```python
from build123d import *

# Parameters (mm, degrees)
F0_R     = 11.949999
F0_R_2   = 5.401318
F1_DEPTH = 25.4
F2_DEPTH = 51.308
F3_R     = 5.08
F4_SIZE  = 5.08


with BuildPart() as f1:
    # F0 (on Front) → F1 (new body)
    with BuildSketch(Plane.XZ):
        with BuildLine():
            ThreePointArc((4.758947, -26.106481), (20.377471, -16.998665), (26.53669, 0))
            ThreePointArc((26.53669, 0), (20.377471, 16.998665), (4.758947, 26.106481))
            ThreePointArc((4.758947, 26.106481), (-26.53669, 0), (4.758947, -26.106481))
        make_face()
        Circle(F0_R, mode=Mode.SUBTRACT)
        with BuildLine():
            ThreePointArc((4.758947, 26.106481), (20.377471, 16.998665), (26.53669, 0))
            ThreePointArc((26.53669, 0), (20.377471, -16.998665), (4.758947, -26.106481))
            Line((4.758947, -26.106481), (78.85573, -12.599387))
            ThreePointArc((78.85573, -12.599387), (63.751977, 0), (78.85573, 12.599387))
            Line((78.85573, 12.599387), (4.758947, 26.106481))
        make_face()
        with BuildLine():
            ThreePointArc((89.366002, 0), (86.393468, 8.203815), (78.85573, 12.599387))
            ThreePointArc((78.85573, 12.599387), (63.751977, 0), (78.85573, -12.599387))
            ThreePointArc((78.85573, -12.599387), (86.393468, -8.203815), (89.366002, 0))
        make_face()
        with Locations((76.55899, 0)):
            Circle(F0_R_2, mode=Mode.SUBTRACT)
    extrude(amount=F1_DEPTH)

    # F0 (on Front) → F2 (join)
    with BuildSketch(Plane.XZ):
        with BuildLine():
            ThreePointArc((4.758947, -26.106481), (20.377471, -16.998665), (26.53669, 0))
            ThreePointArc((26.53669, 0), (20.377471, 16.998665), (4.758947, 26.106481))
            ThreePointArc((4.758947, 26.106481), (-26.53669, 0), (4.758947, -26.106481))
        make_face()
        Circle(F0_R, mode=Mode.SUBTRACT)
    extrude(amount=F2_DEPTH)

    # F3
    f3_edges = [f1.edges().sort_by_distance(p)[0] for p in [
        (-4.758947, -51.308, 26.106481),
        (-11.949999, -51.308, 0),
    ]]
    fillet(f3_edges, radius=F3_R)

    # F4
    f4_edges = [f1.edges().sort_by_distance(p)[0] for p in [
        (71.157671, -25.4, 0),
    ]]
    chamfer(f4_edges, length=F4_SIZE)


solid = f1.part
```
Read the model definition and answer for the solid it produces. Units are mm, in the model's axes. Coordinates: 2 decimals unless noted, no trailing zeros. Write each loop counter-clockwise with the first axis right and the second up, starting at its lowest first coordinate (ties: lowest second). Pieces come first, ordered by that corner, then holes. Notation, with made-up numbers: (69, -15) -> (121, -15) arc R26 ccw to (121, -1) -> close; hole circle Ø5 at (78.25, 41.5). An arc over 180 degrees is marked (long way). Write item = value, one per line.
(1) Section C-C on x = 53.5 is taken. Write down the section's boundary in (y, z).
From the geometry:
outline = (-25.4, -17.22) -> (0, -17.22) -> (0, 17.22) -> (-25.4, 17.22) -> close
(2) Section A-A on y = -38 is taken. Write down the section's boundary in (x, z), plus the area to 3 significant figures.
From the geometry:
outline = circle Ø53.07 at (0, 0); hole circle Ø23.9 at (0, 0)
area = 1,760 mm2
(3) For a pull along X with two mould halves and no side action, classify faces 1 (the face through (5.514, -22.79, -10.602)), 2 (the face through (42.326, -12.522, 19.258)), 3 (the face through (46, -25.4, 0)) as +X half, -X half, draft (parallel to the pull), parting line (faces both ways), or undercut.
From the geometry:
face_1 = undercut
face_2 = +X half
face_3 = draft
(4) Given pin 1 Ø3 at (x, y) = (41.5, -21) entering from +Z; pin 2 Ø12 at (y, z) = (-39.5, 3.5) entering from -X; pin 3 Ø5 at (y, z) = (-9.5, 12.5) entering from +X, each flat-ended and moving along its own axis, determine where each tip first touches the part or whether it passes through.
From the geometry:
pin_1 = 19.68
pin_2 = -26.54
pin_3 = 84.56
(5) Section B-B on z = -3 is taken. Count the separate pieces of the cut face and the enclosed holes in it, plus the area to 3 significant figures.
From the geometry:
separate_pieces = 3
enclosed_holes = 0
area = 2,830 mm2
(6) Straight lines are drawn through the part: L1, parallel to Z at x = -0.5, y = -19; L2, parallel to Y at x = 62, z = -13; L3, parallel to Z at x = -1, y = -49. For each, find the intervals that lie inside material, in ascending order. Write a range as from..to.
From the geometry:
L1 = -26.53..-11.94, 11.94..26.53
L2 = -25.4..0
L3 = -25.69..-12.73, 12.73..25.69
